Here's how the part is built. I have some questions about the finished solid (model axes, mm). A direction names the side the tool comes from. Coordinates: 2 decimals unless noted, no trailing zeros. Order: outer loops, then holes, each group sorted by start corner. A loop starts at its lowest first (then second) coordinate and runs counter-clockwise, first axis right, second up. Notation, with made-up numbers: (-9.75, 55) - (28.25, 55) arc R16 ccw to (28.25, 67) - close; hole circle Ø8 at (10, 39). An arc over 180 degrees is marked (long way). Use one line per item in the form item = value. Start each with the question number.
from build123d import *

# Parameters (mm, degrees)
SKETCH1_W           = 27
SKETCH1_H           = 22
SKETCH1_R           = 8
BOSS_EXTRUDE1_DEPTH = 5
SKETCH2_W           = 5
SKETCH2_H           = 7
BOSS_EXTRUDE2_DEPTH = 7
SKETCH3_R           = 1
CUT_EXTRUDE1_DEPTH  = 26.3
FILLET1_R           = 1
SKETCH4_R           = 1
CUT_EXTRUDE2_DEPTH  = 23


with BuildPart() as part:
    # Sketch1 → Boss-Extrude1 (new body)
    with BuildSketch(Plane.XY):
        Rectangle(SKETCH1_W, SKETCH1_H)
        Circle(SKETCH1_R, mode=Mode.SUBTRACT)
    extrude(amount=BOSS_EXTRUDE1_DEPTH)

    # Sketch2 → Boss-Extrude2 (add)
    with BuildSketch(Plane.XY.offset(5)):
        with Locations((-9.3, -7.5)):
            Rectangle(SKETCH2_W, SKETCH2_H)
        with Locations((9.3, -7.5)):
            Rectangle(SKETCH2_W, SKETCH2_H)
    extrude(amount=BOSS_EXTRUDE2_DEPTH)

    # Sketch3 → Cut-Extrude1 (cut, through all)
    with BuildSketch(Plane.ZY.offset(11.8)):
        with Locations((8.386176527, -7.561390553)):
            Circle(SKETCH3_R)
    extrude(amount=-CUT_EXTRUDE1_DEPTH, mode=Mode.SUBTRACT)

    # Fillet1
    fillet1_edges = [part.edges().sort_by_distance(p)[0] for p in [
        (-9.3, -11, 12),
        (-9.3, -4, 12),
        (9.3, -11, 12),
        (9.3, -4, 12),
    ]]
    fillet(fillet1_edges, radius=FILLET1_R)

    # Sketch4 → Cut-Extrude2 (cut, through all)
    with BuildSketch(Plane(origin=(0, 11, 0), x_dir=(1, 0, 0), z_dir=(0, 1, 0))):
        with Locations((-11, -1.944370678)):
            Circle(SKETCH4_R)
        with Locations((11, -1.944370678)):
            Circle(SKETCH4_R)
    extrude(amount=-CUT_EXTRUDE2_DEPTH, mode=Mode.SUBTRACT)


solid = part.part
1) Suppose I cut it at D-D, the plane z = 2.5. List the corners of the cut face in (x, y) for me.
2) For pin 1 (2 mm diameter, centred on y = -9, z = 8, fed in from +X); pin 2 (5.5 mm diameter, centred on x = -3, y = -7, fed in from +Z); pin 3 (5.5 mm diameter, centred on y = -7.5, z = 8, fed in from -X), each with a flat end and sliding along its axis, tell me the tip position at first contact or that it passes through.
3) Which directions (+Z, -Z, +X, -X, +Y, -Y) give clear straight access to the entire face, cutting with the end or side of a thin tool? Please do faces 1 (the flat face through (9, -4, 8)), 2 (the flat face through (-11.8, -6.77, 9.23)), 3 (the cylindrical face through (10, 0, 2)), 4 (the flat face through (0, -9, 5)).
4) Suppose I cut it at C-C, the plane y = 0. List the corners of the cut face in (x, z) for me, then the cut area to 3 significant figures.
5) If we mould it in two halves opening along X, with no side actions, what happens to faces 5 (the flat face through (6.8, -6.77, 9.23)), 6 (the flat face through (11.8, -6.77, 9.23)), 7 (the flat face through (-3.2, 7.5, 0))? For each: pulls with the +X half, pulls with the -X half, needs draft (parallel to the pull), parting line crosses it, or undercut.
6) Suppose I cut it at A-A, the plane z = 5.5. List the corners of the cut face in (x, y) for me.
7) I need wall thicknesses on probe 1 along X at (y, z) = (-8, 9.5); probe 2 along Y at (x, z) = (-4, 2.5); probe 3 along Y at (x, z) = (10.25, 8.5). Which ranges of each line are inside material? Lowest first, please. Write a range as [from, to].
8) Suppose I cut it at B-B, the plane x = -11.5. List the corners of the cut face in (y, z) for me, then the cut area to 3 significant figures.
From the geometry:
q1.outline = (-13.5, -11) - (-11.83, -11) - (-11.83, 11) - (-13.5, 11) - close; (-10.17, -11) - (10.17, -11) - (10.17, 11) - (-10.17, 11) - close; (11.83, -11) - (13.5, -11) - (13.5, 11) - (11.83, 11) - close; hole circle Ø16 at (0, 0)
q2.pin_1 = 11.8
q2.pin_2 = 5
q2.pin_3 = -11.8
q3.face_1 = +Z, +X, -X, +Y
q3.face_2 = +Z, -X, +Y, -Y
q3.face_3 = +Y, -Y
q3.face_4 = +Z, +Y, -Y
q4.outline = (-13.5, 0) - (-8, 0) - (-8, 5) - (-13.5, 5) - close; (8, 0) - (13.5, 0) - (13.5, 5) - (8, 5) - close; hole circle Ø2 at (-11, 1.94); hole circle Ø2 at (11, 1.94)
q4.area = 48.7 mm2
q5.face_5 = undercut
q5.face_6 = pulls with the +X half
q5.face_7 = needs draft
q6.outline = (-11.8, -11) - (-6.8, -11) - (-6.8, -4) - (-11.8, -4) - close; (6.8, -11) - (11.8, -11) - (11.8, -4) - (6.8, -4) - close
q7.probe_1 = [-11.8, -6.8], [6.8, 11.8]
q7.probe_2 = [-11, -6.93], [6.93, 11]
q7.probe_3 = [-11, -8.55], [-6.57, -4]
q8.outline = (-11, 0) - (11, 0) - (11, 1.08) - (-11, 1.08) - close; (-11, 2.81) - (11, 2.81) - (11, 5) - (-4, 5) - (-4, 11) arc R1 ccw to (-5, 12) - (-10, 12) arc R1 ccw to (-11, 11) - close; hole circle Ø2 at (-7.56, 8.39)
q8.area = 117 mm2
